Could you check a few things on this model? Use its own coordinates, in mm. A direction names the side the tool comes from. Give positions to 0.01 mm unless a question says otherwise; leave off trailing zeros.
from build123d import *

# Parameters (mm, degrees)
F0_W     = 85.4
F0_H     = 127.8
F1_DEPTH = 52
F2_W     = 85.4
F2_H     = 127.8
F2_R     = 3.5
F3_DEPTH = 19
F4_R     = 3


with BuildPart() as f1:
    # F0 (on Top) → F1 (new body)
    with BuildSketch(Plane.XY):
        Rectangle(F0_W, F0_H)
    extrude(amount=F1_DEPTH)

    # F2 (on face) → F3 (cut)
    with BuildSketch(Plane.XY.offset(52)):
        Rectangle(F2_W, F2_H)
        with Locations((-31.54, -49.48)):
            Circle(F2_R, mode=Mode.SUBTRACT)
        with Locations((-22.54, -49.48)):
            Circle(F2_R, mode=Mode.SUBTRACT)
        with Locations((-31.54, -40.48)):
            Circle(F2_R, mode=Mode.SUBTRACT)
        with Locations((-22.54, -40.48)):
            Circle(F2_R, mode=Mode.SUBTRACT)
        with Locations((-13.54, -49.48)):
            Circle(F2_R, mode=Mode.SUBTRACT)
        with Locations((-4.54, -49.48)):
            Circle(F2_R, mode=Mode.SUBTRACT)
        with Locations((-13.54, -40.48)):
            Circle(F2_R, mode=Mode.SUBTRACT)
        with Locations((-4.54, -40.48)):
            Circle(F2_R, mode=Mode.SUBTRACT)
        with Locations((-31.54, -31.48)):
            Circle(F2_R, mode=Mode.SUBTRACT)
        with Locations((-22.54, -31.48)):
            Circle(F2_R, mode=Mode.SUBTRACT)
        with Locations((-31.54, -22.48)):
            Circle(F2_R, mode=Mode.SUBTRACT)
        with Locations((-22.54, -22.48)):
            Circle(F2_R, mode=Mode.SUBTRACT)
        with Locations((-31.54, -13.48)):
            Circle(F2_R, mode=Mode.SUBTRACT)
        with Locations((-22.54, -13.48)):
            Circle(F2_R, mode=Mode.SUBTRACT)
        with Locations((-31.54, -4.48)):
            Circle(F2_R, mode=Mode.SUBTRACT)
        with Locations((-22.54, -4.48)):
            Circle(F2_R, mode=Mode.SUBTRACT)
        with Locations((-13.54, -31.48)):
            Circle(F2_R, mode=Mode.SUBTRACT)
        with Locations((-13.54, -22.48)):
            Circle(F2_R, mode=Mode.SUBTRACT)
        with Locations((-4.54, -31.48)):
            Circle(F2_R, mode=Mode.SUBTRACT)
        with Locations((-4.54, -22.48)):
            Circle(F2_R, mode=Mode.SUBTRACT)
        with Locations((-13.54, -13.48)):
            Circle(F2_R, mode=Mode.SUBTRACT)
        with Locations((-13.54, -4.48)):
            Circle(F2_R, mode=Mode.SUBTRACT)
        with Locations((-4.54, -13.48)):
            Circle(F2_R, mode=Mode.SUBTRACT)
        with Locations((-4.54, -4.48)):
            Circle(F2_R, mode=Mode.SUBTRACT)
        with Locations((4.46, -49.48)):
            Circle(F2_R, mode=Mode.SUBTRACT)
        with Locations((13.46, -49.48)):
            Circle(F2_R, mode=Mode.SUBTRACT)
        with Locations((4.46, -40.48)):
            Circle(F2_R, mode=Mode.SUBTRACT)
        with Locations((13.46, -40.48)):
            Circle(F2_R, mode=Mode.SUBTRACT)
        with Locations((22.46, -49.48)):
            Circle(F2_R, mode=Mode.SUBTRACT)
        with Locations((31.46, -49.48)):
            Circle(F2_R, mode=Mode.SUBTRACT)
        with Locations((22.46, -40.48)):
            Circle(F2_R, mode=Mode.SUBTRACT)
        with Locations((31.46, -40.48)):
            Circle(F2_R, mode=Mode.SUBTRACT)
        with Locations((4.46, -31.48)):
            Circle(F2_R, mode=Mode.SUBTRACT)
        with Locations((4.46, -22.48)):
            Circle(F2_R, mode=Mode.SUBTRACT)
        with Locations((13.46, -31.48)):
            Circle(F2_R, mode=Mode.SUBTRACT)
        with Locations((13.46, -22.48)):
            Circle(F2_R, mode=Mode.SUBTRACT)
        with Locations((4.46, -13.48)):
            Circle(F2_R, mode=Mode.SUBTRACT)
        with Locations((4.46, -4.48)):
            Circle(F2_R, mode=Mode.SUBTRACT)
        with Locations((13.46, -13.48)):
            Circle(F2_R, mode=Mode.SUBTRACT)
        with Locations((13.46, -4.48)):
            Circle(F2_R, mode=Mode.SUBTRACT)
        with Locations((22.46, -31.48)):
            Circle(F2_R, mode=Mode.SUBTRACT)
        with Locations((31.46, -31.48)):
            Circle(F2_R, mode=Mode.SUBTRACT)
        with Locations((22.46, -22.48)):
            Circle(F2_R, mode=Mode.SUBTRACT)
        with Locations((31.46, -22.48)):
            Circle(F2_R, mode=Mode.SUBTRACT)
        with Locations((22.46, -13.48)):
            Circle(F2_R, mode=Mode.SUBTRACT)
        with Locations((31.46, -13.48)):
            Circle(F2_R, mode=Mode.SUBTRACT)
        with Locations((22.46, -4.48)):
            Circle(F2_R, mode=Mode.SUBTRACT)
        with Locations((31.46, -4.48)):
            Circle(F2_R, mode=Mode.SUBTRACT)
        with Locations((-31.54, 4.52)):
            Circle(F2_R, mode=Mode.SUBTRACT)
        with Locations((-22.54, 4.52)):
            Circle(F2_R, mode=Mode.SUBTRACT)
        with Locations((-31.54, 13.52)):
            Circle(F2_R, mode=Mode.SUBTRACT)
        with Locations((-22.54, 13.52)):
            Circle(F2_R, mode=Mode.SUBTRACT)
        with Locations((-31.54, 22.52)):
            Circle(F2_R, mode=Mode.SUBTRACT)
        with Locations((-22.54, 22.52)):
            Circle(F2_R, mode=Mode.SUBTRACT)
        with Locations((-31.54, 31.52)):
            Circle(F2_R, mode=Mode.SUBTRACT)
        with Locations((-22.54, 31.52)):
            Circle(F2_R, mode=Mode.SUBTRACT)
        with Locations((-13.54, 4.52)):
            Circle(F2_R, mode=Mode.SUBTRACT)
        with Locations((-13.54, 13.52)):
            Circle(F2_R, mode=Mode.SUBTRACT)
        with Locations((-4.54, 4.52)):
            Circle(F2_R, mode=Mode.SUBTRACT)
        with Locations((-4.54, 13.52)):
            Circle(F2_R, mode=Mode.SUBTRACT)
        with Locations((-13.54, 22.52)):
            Circle(F2_R, mode=Mode.SUBTRACT)
        with Locations((-13.54, 31.52)):
            Circle(F2_R, mode=Mode.SUBTRACT)
        with Locations((-4.54, 22.52)):
            Circle(F2_R, mode=Mode.SUBTRACT)
        with Locations((-4.54, 31.52)):
            Circle(F2_R, mode=Mode.SUBTRACT)
        with Locations((-31.54, 40.52)):
            Circle(F2_R, mode=Mode.SUBTRACT)
        with Locations((-22.54, 40.52)):
            Circle(F2_R, mode=Mode.SUBTRACT)
        with Locations((-31.54, 49.52)):
            Circle(F2_R, mode=Mode.SUBTRACT)
        with Locations((-22.54, 49.52)):
            Circle(F2_R, mode=Mode.SUBTRACT)
        with Locations((-13.54, 40.52)):
            Circle(F2_R, mode=Mode.SUBTRACT)
        with Locations((-4.54, 40.52)):
            Circle(F2_R, mode=Mode.SUBTRACT)
        with Locations((-13.54, 49.52)):
            Circle(F2_R, mode=Mode.SUBTRACT)
        with Locations((-4.54, 49.52)):
            Circle(F2_R, mode=Mode.SUBTRACT)
        with Locations((4.46, 4.52)):
            Circle(F2_R, mode=Mode.SUBTRACT)
        with Locations((4.46, 13.52)):
            Circle(F2_R, mode=Mode.SUBTRACT)
        with Locations((13.46, 4.52)):
            Circle(F2_R, mode=Mode.SUBTRACT)
        with Locations((13.46, 13.52)):
            Circle(F2_R, mode=Mode.SUBTRACT)
        with Locations((4.46, 22.52)):
            Circle(F2_R, mode=Mode.SUBTRACT)
        with Locations((4.46, 31.52)):
            Circle(F2_R, mode=Mode.SUBTRACT)
        with Locations((13.46, 22.52)):
            Circle(F2_R, mode=Mode.SUBTRACT)
        with Locations((13.46, 31.52)):
            Circle(F2_R, mode=Mode.SUBTRACT)
        with Locations((22.46, 4.52)):
            Circle(F2_R, mode=Mode.SUBTRACT)
        with Locations((31.46, 4.52)):
            Circle(F2_R, mode=Mode.SUBTRACT)
        with Locations((22.46, 13.52)):
            Circle(F2_R, mode=Mode.SUBTRACT)
        with Locations((31.46, 13.52)):
            Circle(F2_R, mode=Mode.SUBTRACT)
        with Locations((22.46, 22.52)):
            Circle(F2_R, mode=Mode.SUBTRACT)
        with Locations((31.46, 22.52)):
            Circle(F2_R, mode=Mode.SUBTRACT)
        with Locations((22.46, 31.52)):
            Circle(F2_R, mode=Mode.SUBTRACT)
        with Locations((31.46, 31.52)):
            Circle(F2_R, mode=Mode.SUBTRACT)
        with Locations((4.46, 40.52)):
            Circle(F2_R, mode=Mode.SUBTRACT)
        with Locations((13.46, 40.52)):
            Circle(F2_R, mode=Mode.SUBTRACT)
        with Locations((4.46, 49.52)):
            Circle(F2_R, mode=Mode.SUBTRACT)
        with Locations((13.46, 49.52)):
            Circle(F2_R, mode=Mode.SUBTRACT)
        with Locations((22.46, 40.52)):
            Circle(F2_R, mode=Mode.SUBTRACT)
        with Locations((31.46, 40.52)):
            Circle(F2_R, mode=Mode.SUBTRACT)
        with Locations((22.46, 49.52)):
            Circle(F2_R, mode=Mode.SUBTRACT)
        with Locations((31.46, 49.52)):
            Circle(F2_R, mode=Mode.SUBTRACT)
    extrude(amount=-F3_DEPTH, mode=Mode.SUBTRACT)

    # F4
    f4_edges = [f1.edges().sort_by_distance(p)[0] for p in [
        (-42.7, 63.9, 16.5),
        (-42.7, -63.9, 16.5),
        (42.7, -63.9, 16.5),
        (42.7, 63.9, 16.5),
    ]]
    fillet(f4_edges, radius=F4_R)


solid = f1.part
Item 1: Please list where this line runs through material, in increasing order: line 1 along Z through (x, y) = (-36, 8).
Findings:
line 1: z = 0 to 33
Item 2: For faces 3 (the cylindrical face through (1.683, -15.61, 42.633)), 4 (the flat face through (-14, -49, 52)), which set-ups out of +Z, -Z, +X, -X, +Y, -Y let a thin tool reach every point of the face, with its end or its side?
Findings:
face 3: +Z
face 4: +Z, +X, -X, +Y, -Y
Item 3: We'd pull the mould along Y, two halves only. Please class faces 1 (the flat face through (31, 14, 52)), 2 (the cylindrical face through (-28.2, -30.43, 42.63)): +Y half, -Y half, draft (parallel to the pull), parting line (faces both ways), or undercut.
Findings:
face 1: draft
face 2: undercut
Item 4: Imagine slicing it at A-A on z = 40. Give the number of separate pieces and of enclosed holes in the cut face, then the cut area to 3 significant figures.
Findings:
separate pieces: 96
enclosed holes: 0
area: 3,690 mm2
